Could you check a few things on this drawing? It's one solid part, dimensions in mm from its lowest x, y, z. A direction names the side the tool comes from. Give positions to 0.01 mm unless a question says otherwise; leave off trailing zeros. Order: outer loops, then holes, each group sorted by start corner. A loop starts at its lowest first (then second) coordinate and runs counter-clockwise, first axis right, second up.
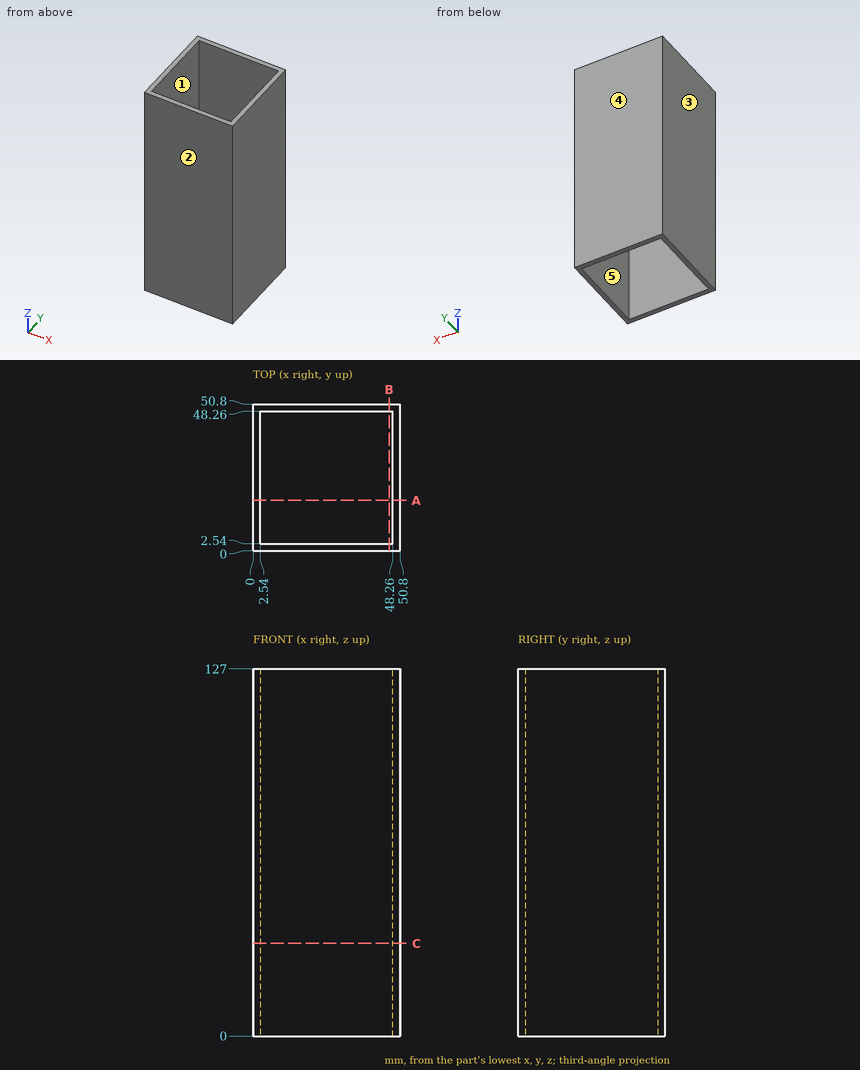
Q1. Thinking about a two-plate mould opening in Y: for the marked faces 1, 2 and 3, which applies, released by +Y, released by -Y, zero draft, split by the parting line, or undercut?
Filled sheet:
face 1: undercut
face 2: released by -Y
face 3: zero draft
Q2. For the marked faces 4 and 5, which set-ups out of +Z, -Z, +X, -X, +Y, -Y let a thin tool reach every point of the face, with its end or its side?
Filled sheet:
face 4: +Z, -Z, +X, -X, +Y
face 5: +Z, -Z
Q3. I need wall thicknesses on L1, parallel to Y at x = 16.5, z = 70.5. Which ranges of the line are inside material? Lowest first, please.
Filled sheet:
L1: y = 0 to 2.54, 48.26 to 50.8
Q4. If we section it at C-C on z = 32: List the corners of the cut face in (x, y) for me.
Filled sheet:
outline: (0, 0) - (50.8, 0) - (50.8, 50.8) - (0, 50.8) - close; hole (2.54, 2.54) - (48.26, 2.54) - (48.26, 48.26) - (2.54, 48.26) - close
Q5. If we section it at A-A on y = 17.5: List the corners of the cut face in (x, z) for me, plus the area to 3 significant figures.
Filled sheet:
outline: (0, 0) - (2.54, 0) - (2.54, 127) - (0, 127) - close; (48.26, 0) - (50.8, 0) - (50.8, 127) - (48.26, 127) - close
area: 645 mm2
Q6. I'm going to push flat-ended pins straight in: P1, Ø5, axis at x = 45.5, y = 30, coming from the +Z side; P2, Ø3, axis at y = 16.5, z = 25, coming from the -X side. Where does each tip first touch, or does it pass through?
Filled sheet:
P1: passes through
P2: stops at x = 0
